```python
from build123d import *

# Parameters (mm, degrees)
BOSS_EXTRUDE1_DEPTH      = 250
BOSS_EXTRUDE2_DEPTH      = 10
BOSS_EXTRUDE2_DEPTH_BACK = 20
SKETCH2_R                = 12.5
SKETCH3_R                = 8.5
CUT_EXTRUDE1_DEPTH       = 253.586618806
BOSS_EXTRUDE3_DEPTH      = 10
BOSS_EXTRUDE3_DEPTH_BACK = 20
SKETCH4_R                = 17.5
SKETCH5_R                = 12.5
CUT_EXTRUDE2_DEPTH       = 271.335439778
CUT_EXTRUDE3_START       = 12.5
SKETCH6_W                = 5
SKETCH6_H                = 40
CUT_EXTRUDE3_DEPTH       = 39


with BuildPart() as part:
    # Sketch1 → Boss-Extrude1 (new body)
    with BuildSketch(Plane(origin=(0, 0, 0), x_dir=(1, 0, 0), z_dir=(0, 1, 0))):
        Polygon((0, 0), (0, 15), (-5, 15), (-5, 20), (15, 20), (15, 15), (10, 15), (10, 0), (15, 0), (15, -5), (-5, -5), (-5, 0), align=None)
    extrude(amount=BOSS_EXTRUDE1_DEPTH)

    # Sketch2 → Boss-Extrude2 (add, two sides: drawn at the far end of the back side and taken through both)
    with BuildSketch(Plane(origin=(10, 0, 0), x_dir=(0, 0, -1), z_dir=(1, 0, 0)).offset(-BOSS_EXTRUDE2_DEPTH_BACK)):
        with Locations((7.5, 0)):
            Circle(SKETCH2_R)
    extrude(amount=BOSS_EXTRUDE2_DEPTH + BOSS_EXTRUDE2_DEPTH_BACK)

    # Sketch3 → Cut-Extrude1 (cut, through all)
    with BuildSketch(Plane(origin=(20, 0, 0), x_dir=(0, 0, -1), z_dir=(1, 0, 0))):
        with Locations((7.5, 0)):
            Circle(SKETCH3_R)
    extrude(amount=-CUT_EXTRUDE1_DEPTH, mode=Mode.SUBTRACT)

    # Sketch4 → Boss-Extrude3 (add, two sides: drawn at the far end of the back side and taken through both)
    with BuildSketch(Plane.ZY.offset(-BOSS_EXTRUDE3_DEPTH_BACK)):
        with Locations((-7.5, 250)):
            Circle(SKETCH4_R)
    extrude(amount=BOSS_EXTRUDE3_DEPTH + BOSS_EXTRUDE3_DEPTH_BACK)

    # Sketch5 → Cut-Extrude2 (cut, through all)
    with BuildSketch(Plane(origin=(20, 0, 0), x_dir=(0, 0, -1), z_dir=(1, 0, 0))):
        with Locations((7.5, 250)):
            Circle(SKETCH5_R)
    extrude(amount=-CUT_EXTRUDE2_DEPTH, mode=Mode.SUBTRACT)

    # Sketch6 → Cut-Extrude3 (cut)
    with BuildSketch(Plane(origin=(0, 0, 0), x_dir=(1, 0, 0), z_dir=(0, 1, 0)).offset(CUT_EXTRUDE3_START)):
        with Locations((5, 5)):
            Rectangle(SKETCH6_W, SKETCH6_H)
    extrude(amount=-CUT_EXTRUDE3_DEPTH, mode=Mode.SUBTRACT)


solid = part.part
```
Can you work these out from the model? Positions are in its coordinate system, mm. A direction names the side the tool comes from. Round coordinates to 2 decimals unless told otherwise and drop trailing zeros. Loops run counter-clockwise (first coordinate to the right, second up) from the corner with the lowest first, then second, coordinate; pieces in that order, holes last. Notation, with made-up numbers: M 22,79 L 38,79 A34 ccw 38,111 Z; hole C 38,47 d6. An arc over 180 degrees is marked long. Answer in a Markdown table with one row per item.
1. If we section it at D-D, the plane y = 154: Please give me the cut outline in (x, z), plus the area to 3 significant figures.
Established:
| item | result |
|---|---|
| outline | M -5,-20 L 15,-20 L 15,-15 L 10,-15 L 10,0 L 15,0 L 15,5 L -5,5 L -5,0 L 0,0 L 0,-15 L -5,-15 Z |
| area | 350 mm² |
2. If we section it at A-A, the plane y = 250: Please give me the cut outline in (x, z).
Established:
| item | result |
|---|---|
| outline | M -10,-25 L 20,-25 L 20,-20 L -10,-20 Z; M -10,5 L 20,5 L 20,10 L -10,10 Z |
3. Thinking about a two-plate mould opening in X: for faces 5 (the face through (12, 121, 0)), 6 (the face through (7.5, 9, -7)), 7 (the face through (-5, 117, -17)), 8 (the face through (2.5, 9, -7)), which applies, pulls with the +X half, pulls with the -X half, needs draft (parallel to the pull), parting line crosses it, or undercut?
Established:
| item | result |
|---|---|
| face 5 | needs draft |
| face 6 | undercut |
| face 7 | pulls with the -X half |
| face 8 | undercut |
4. If we section it at C-C, the plane x = 17.5: Please give me the cut outline in (y, z).
Established:
| item | result |
|---|---|
| outline | C 0,-7.5 d25; C 250,-7.5 d35; hole C 0,-7.5 d17; hole C 250,-7.5 d25 |
5. On a 3-axis mill with a long thin cutter (end or side, diameter ignored), from which of +Z, -Z, +X, -X, +Y, -Y can I reach the whole of each face in a straight line? I mean faces 1 (the face through (13, 121, -15)), 2 (the face through (-3, 121, 0)), 3 (the face through (5, 117, -20)), 4 (the face through (5, 117, 5)). Say none if no direction works.
Established:
| item | result |
|---|---|
| face 1 | +X |
| face 2 | -X |
| face 3 | -Z, +X, -X, -Y |
| face 4 | +Z, +X, -X, -Y |
6. Please list where these lines run through material, in increasing order: line 1 (Y direction, x = -4.5, z = -7.5); line 2 (Y direction, x = 15, z = -14); line 3 (Z direction, x = -0.25, y = 145). Write a range as from..to.
Established:
| item | result |
|---|---|
| line 1 | -12.5..-8.5, 8.5..12.5, 232.5..237.5, 262.5..267.5 |
| line 2 | -10.68..-5.48, 5.48..10.68, 233.75..239.32, 260.68..266.25 |
| line 3 | -20..-15, 0..5 |
7. If we section it at B-B, the plane z = -7.5: Please give me the cut outline in (x, y), plus the area to 3 significant figures.
Established:
| item | result |
|---|---|
| outline | M -10,-12.5 L 2.5,-12.5 L 2.5,-8.5 L -10,-8.5 Z; M -10,8.5 L 2.5,8.5 L 2.5,12.5 L 7.5,12.5 L 7.5,8.5 L 20,8.5 L 20,12.5 L 10,12.5 L 10,232.5 L 20,232.5 L 20,237.5 L -10,237.5 L -10,232.5 L 0,232.5 L 0,12.5 L -10,12.5 Z; M -10,262.5 L 20,262.5 L 20,267.5 L -10,267.5 Z; M 7.5,-12.5 L 20,-12.5 L 20,-8.5 L 7.5,-8.5 Z |
| area | 2,700 mm² |
8. I'm going to push flat-ended pins straight in: pin 1 Ø2.5 at (x, y) = (-3.5, 88.5) entering from +Z; pin 2 Ø1.5 at (y, z) = (224, 3) entering from +X; pin 3 Ø5 at (x, y) = (1.5, 116) entering from -Z; pin 4 Ø15 at (y, z) = (250, -7.5) entering from +X. Where does each tip first touch, or does it pass through?
Established:
| item | result |
|---|---|
| pin 1 | z = 5 |
| pin 2 | x = 15 |
| pin 3 | z = -20 |
| pin 4 | through |
